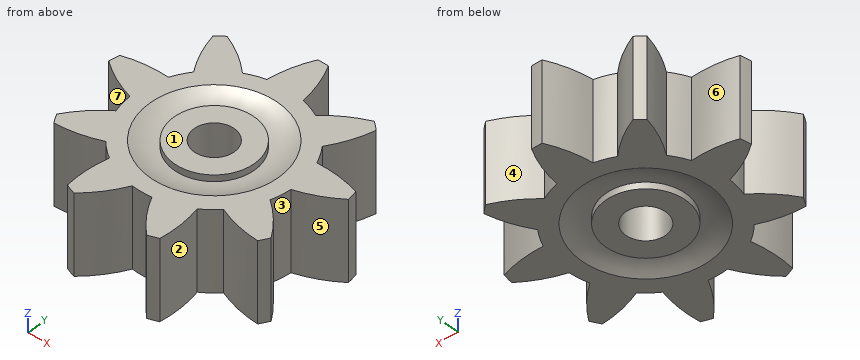
```python
from build123d import *

# Parameters (mm, degrees)
F0_R     = 4.7625
F0_R_2   = 3.175
F0_R_3   = 1.5875
F1_DEPTH = 3.175
F2_R     = 5.08
F2_R_2   = 3.175
F3_DEPTH = 0.508
F4_R     = 5.08
F4_R_2   = 3.175
F5_DEPTH = 0.508


# Not quite as in the source:
# - a fillet or chamfer that OpenCascade refuses, or shapes differently, is made with other operations: its cross-section is extruded or revolved along the edge and cut away or added


with BuildPart() as f1:
    # F0 (on Top) → F1 (new body, symmetric)
    with BuildSketch(Plane.XY):
        with BuildLine():
            ThreePointArc((6.3411298165, -0.3355184801), (6.3477820668, -0.1678178556), (6.35, 0))
            ThreePointArc((6.35, 0), (6.222203729, 1.2675491134), (5.8439588173, 2.4840783686))
            ThreePointArc((5.8439588173, 2.4840783686), (5.499261314, 3.175), (5.0732543809, 3.8189776102))
            ThreePointArc((5.0732543809, 3.8189776102), (4.0817013215, 4.8643822138), (2.879997381, 5.6593387498))
            ThreePointArc((2.879997381, 5.6593387498), (2.1718279101, 5.967048142), (1.4315468375, 6.1865316335))
            ThreePointArc((1.4315468375, 6.1865316335), (0, 6.35), (-1.4315468375, 6.1865316335))
            ThreePointArc((-1.4315468375, 6.1865316335), (-2.1718279101, 5.967048142), (-2.879997381, 5.6593387498))
            ThreePointArc((-2.879997381, 5.6593387498), (-4.0817013215, 4.8643822138), (-5.0732543809, 3.8189776102))
            ThreePointArc((-5.0732543809, 3.8189776102), (-5.499261314, 3.175), (-5.8439588173, 2.4840783686))
            ThreePointArc((-5.8439588173, 2.4840783686), (-6.2535292316, 1.1026659282), (-6.3411298165, -0.3355184801))
            ThreePointArc((-6.3411298165, -0.3355184801), (-6.2535292316, -1.1026659282), (-6.0734669747, -1.8535098888))
            ThreePointArc((-6.0734669747, -1.8535098888), (-5.499261314, -3.175), (-4.6419201372, -4.3330217447))
            ThreePointArc((-4.6419201372, -4.3330217447), (-4.0817013215, -4.8643822138), (-3.4611324355, -5.3238202697))
            ThreePointArc((-3.4611324355, -5.3238202697), (-2.1718279101, -5.967048142), (-0.7707044365, -6.3030559788))
            ThreePointArc((-0.7707044365, -6.3030559788), (0, -6.35), (0.7707044365, -6.3030559788))
            ThreePointArc((0.7707044365, -6.3030559788), (2.1718279101, -5.967048142), (3.4611324355, -5.3238202697))
            ThreePointArc((3.4611324355, -5.3238202697), (4.0817013215, -4.8643822138), (4.6419201372, -4.3330217447))
            ThreePointArc((4.6419201372, -4.3330217447), (5.499261314, -3.175), (6.0734669747, -1.8535098888))
            ThreePointArc((6.0734669747, -1.8535098888), (6.2535292316, -1.1026659282), (6.3411298165, -0.3355184801))
        make_face()
        Circle(F0_R, mode=Mode.SUBTRACT)
        Circle(F0_R)
        Circle(F0_R_2, mode=Mode.SUBTRACT)
        Circle(F0_R_2)
        Circle(F0_R_3, mode=Mode.SUBTRACT)
        with BuildLine():
            ThreePointArc((5.8439588173, 2.4840783686), (6.222203729, 1.2675491134), (6.35, 0))
            ThreePointArc((6.35, 0), (6.3477820668, -0.1678178556), (6.3411298165, -0.3355184801))
            ThreePointArc((6.3411298165, -0.3355184801), (7.9650557648, 0.3109444224), (9.4435123046, 1.2432619809))
            ThreePointArc((9.4435123046, 1.2432619809), (9.3802938474, 1.6539988923), (9.2992194678, 2.0615873228))
            ThreePointArc((9.2992194678, 2.0615873228), (7.5910533822, 2.4320173351), (5.8439588173, 2.4840783686))
        make_face()
        with BuildLine():
            ThreePointArc((2.879997381, 5.6593387498), (4.0817013215, 4.8643822138), (5.0732543809, 3.8189776102))
            ThreePointArc((5.0732543809, 3.8189776102), (5.9017154857, 5.358036403), (6.4349967275, 7.0225666331))
            ThreePointArc((6.4349967275, 7.0225666331), (6.1225519823, 7.2965733207), (5.7984526113, 7.5566905663))
            ThreePointArc((5.7984526113, 7.5566905663), (4.2518136514, 6.7424684237), (2.879997381, 5.6593387498))
        make_face()
        with BuildLine():
            ThreePointArc((8.448778186, -4.3981555411), (7.3783548704, -3.0164016935), (6.0734669747, -1.8535098888))
            ThreePointArc((6.0734669747, -1.8535098888), (5.499261314, -3.175), (4.6419201372, -4.3330217447))
            ThreePointArc((4.6419201372, -4.3330217447), (6.3014579298, -4.8816419092), (8.0333035214, -5.1177787695))
            ThreePointArc((8.0333035214, -5.1177787695), (8.248891971, -4.7625), (8.448778186, -4.3981555411))
        make_face()
        with BuildLine():
            ThreePointArc((-1.4315468375, 6.1865316335), (0, 6.35), (1.4315468375, 6.1865316335))
            ThreePointArc((1.4315468375, 6.1865316335), (1.0768969406, 7.8980436026), (0.4154746647, 9.5159343106))
            ThreePointArc((0.4154746647, 9.5159343106), (0, 9.525), (-0.4154746647, 9.5159343106))
            ThreePointArc((-0.4154746647, 9.5159343106), (-1.0768969406, 7.8980436026), (-1.4315468375, 6.1865316335))
        make_face()
        with BuildLine():
            ThreePointArc((3.6450596933, -8.7999525472), (3.7132421134, -7.0534128461), (3.4611324355, -5.3238202697))
            ThreePointArc((3.4611324355, -5.3238202697), (2.1718279101, -5.967048142), (0.7707044365, -6.3030559788))
            ThreePointArc((0.7707044365, -6.3030559788), (1.6893378965, -7.790053738), (2.8642227403, -9.0841539559))
            ThreePointArc((2.8642227403, -9.0841539559), (3.2577418652, -8.950572213), (3.6450596933, -8.7999525472))
        make_face()
        with BuildLine():
            ThreePointArc((-5.0732543809, 3.8189776102), (-4.0817013215, 4.8643822138), (-2.879997381, 5.6593387498))
            ThreePointArc((-2.879997381, 5.6593387498), (-4.2518136514, 6.7424684237), (-5.7984526113, 7.5566905663))
            ThreePointArc((-5.7984526113, 7.5566905663), (-6.1225519823, 7.2965733207), (-6.4349967275, 7.0225666331))
            ThreePointArc((-6.4349967275, 7.0225666331), (-5.9017154857, 5.358036403), (-5.0732543809, 3.8189776102))
        make_face()
        with BuildLine():
            ThreePointArc((-2.8642227403, -9.0841539559), (-1.6893378965, -7.790053738), (-0.7707044365, -6.3030559788))
            ThreePointArc((-0.7707044365, -6.3030559788), (-2.1718279101, -5.967048142), (-3.4611324355, -5.3238202697))
            ThreePointArc((-3.4611324355, -5.3238202697), (-3.7132421134, -7.0534128461), (-3.6450596933, -8.7999525472))
            ThreePointArc((-3.6450596933, -8.7999525472), (-3.2577418652, -8.950572213), (-2.8642227403, -9.0841539559))
        make_face()
        with BuildLine():
            ThreePointArc((-6.3411298165, -0.3355184801), (-6.2535292316, 1.1026659282), (-5.8439588173, 2.4840783686))
            ThreePointArc((-5.8439588173, 2.4840783686), (-7.5910533822, 2.4320173351), (-9.2992194678, 2.0615873228))
            ThreePointArc((-9.2992194678, 2.0615873228), (-9.3802938474, 1.6539988923), (-9.4435123046, 1.2432619809))
            ThreePointArc((-9.4435123046, 1.2432619809), (-7.9650557648, 0.3109444224), (-6.3411298165, -0.3355184801))
        make_face()
        with BuildLine():
            ThreePointArc((-8.0333035214, -5.1177787695), (-6.3014579298, -4.8816419092), (-4.6419201372, -4.3330217447))
            ThreePointArc((-4.6419201372, -4.3330217447), (-5.499261314, -3.175), (-6.0734669747, -1.8535098888))
            ThreePointArc((-6.0734669747, -1.8535098888), (-7.3783548704, -3.0164016935), (-8.448778186, -4.3981555411))
            ThreePointArc((-8.448778186, -4.3981555411), (-8.248891971, -4.7625), (-8.0333035214, -5.1177787695))
        make_face()
    extrude(amount=F1_DEPTH, both=True)

    # F2 (on face) → F3 (cut)
    with BuildSketch(Plane(origin=(0, 0, -3.175), x_dir=(1, 0, 0), z_dir=(0, 0, -1))):
        Circle(F2_R)
        Circle(F2_R_2, mode=Mode.SUBTRACT)
    extrude(amount=-F3_DEPTH, mode=Mode.SUBTRACT)

    # F4 (on face) → F5 (cut)
    with BuildSketch(Plane.XY.offset(3.175)):
        Circle(F4_R)
        Circle(F4_R_2, mode=Mode.SUBTRACT)
    extrude(amount=-F5_DEPTH, mode=Mode.SUBTRACT)

    # F6: fillet of radius 3.81 on 2 edges, made by hand

    # F6_s1 → F6_t2 (revolve)
    with BuildSketch(Plane.XZ):
        with BuildLine():
            ThreePointArc((5.08, 3.175), (4.1629758175, 2.7961903065), (3.1792380475, 2.667))
            Line((3.1792380475, 2.667), (5.08, 2.667))
            Line((5.08, 2.667), (5.08, 3.175))
        make_face()
    revolve(axis=Axis((0, 0, 2.667), (0, 0, 1)))

    # F6_s3 → F6_t4 (revolve)
    with BuildSketch(Plane.XZ):
        with BuildLine():
            ThreePointArc((5.08, -3.175), (4.1629758175, -2.7961903065), (3.1792380475, -2.667))
            Line((3.1792380475, -2.667), (5.08, -2.667))
            Line((5.08, -2.667), (5.08, -3.175))
        make_face()
    revolve(axis=Axis((0, 0, -2.667), (0, 0, -1)))


solid = f1.part
```
Source: CAD feature listing. Evaluate the final solid. Frame: model axes, mm. Face numbers are marked on the shaded views. A direction names the side the tool comes from. Coordinates: 2 decimals unless noted, no trailing zeros. Write each loop counter-clockwise with the first axis right and the second up, starting at its lowest first coordinate (ties: lowest second). Pieces come first, ordered by that corner, then holes. Notation, with made-up numbers: M -6,62 L -1,62 A13 cw -1,67 Z; hole C -16.75,14 d7. An arc over 180 degrees is marked long. Answer as a JSON object with one key per item and string values.
1. Cut plane C-C on y = -6. Output: boundary loops of the cut face in (x, z) (3 decimals).
Evaluation:
{"outline": "M -3.598,-3.175 L 3.598,-3.175 L 3.598,3.175 L -3.598,3.175 Z"}
2. Draft query along Y for the marked faces 1, 2, 3 and 4. Return one class per face: released by +Y, released by -Y, zero draft, split by the parting line, or undercut.
Evaluation:
{"face 1": "zero draft", "face 2": "undercut", "face 3": "undercut", "face 4": "released by +Y"}
3. Ray query, L1, parallel to X at y = -1, z = -1; L2, parallel to Y at x = -6.75, z = 2.75; L3, parallel to Y at x = 7, z = -2.5. Return the intervals inside material, ascending.
Evaluation:
{"L1": "-6.27 to -1.23, 1.23 to 6.27", "L2": "-4.97 to -2.4, -0.2 to 2.5", "L3": "-5.02 to -2.63, -0.11 to 2.49"}
4. Cut plane B-B on x = 7.5. Output: boundary loops of the cut face in (y, z) (3 decimals).
Evaluation:
{"outline": "M -5.079,-3.175 L -3.149,-3.175 L -3.149,3.175 L -5.079,3.175 Z; M 0.09,-3.175 L 2.443,-3.175 L 2.443,3.175 L 0.09,3.175 Z"}
5. Cut plane A-A on x = -6.75. Output: boundary loops of the cut face in (y, z) (3 decimals), plus the area to 3 significant figures.
Evaluation:
{"outline": "M -4.974,-3.175 L -2.403,-3.175 L -2.403,3.175 L -4.974,3.175 Z; M -0.205,-3.175 L 2.497,-3.175 L 2.497,3.175 L -0.205,3.175 Z", "area": "33.5 mm^2"}
6. Contact query for flat-ended pins moving along their axis: P1, Ø4, axis at x = 0, y = 0, coming from the -Z side (3 decimals); P2, Ø2, axis at x = -1.5, z = 1.5, coming from the +Y side; P3, Ø2, axis at y = 0, z = 1.5, coming from the -X side; P4, Ø2, axis at x = 6.5, z = -0.5, coming from the -Y side. Output: stop coordinate, or through.
Evaluation:
{"P1": "z = -3.175", "P2": "y = 9.35", "P3": "x = -9.11", "P4": "y = -5.08"}
7. Access query for the marked faces 5, 6 and 7. Directions: +Z, -Z, +X, -X, +Y, -Y. A direction counts if a zero-diameter tool reaches every point of the face in a straight line with its end or side. Return the directions, or none.
Evaluation:
{"face 5": "+Z, -Z, +X", "face 6": "+Z, -Z", "face 7": "+Z, -Z, -X"}
